```python
from build123d import *

# Parameters (mm, degrees)
RESSALTO_EXTRUS_O1_DEPTH                = 3
BROCA_DE_ROSQUEAR_PARA_TARRAXA_DE_M61_D = 5
ESBO_O4_W                               = 17.804449836
ESBO_O4_H                               = 9.873376728
CORTE_EXTRUS_O1_DEPTH                   = 149.227737241


with BuildPart() as part:
    # Esboço1 → Ressalto-extrusão1 (new body)
    with BuildSketch(Plane.XY):
        Polygon((0, 0), (117.509029813, -27.129097154), (117.509029813, 63.170902846), (0, 90.3), align=None)
    extrude(amount=RESSALTO_EXTRUS_O1_DEPTH)

    # Broca de rosquear para tarraxa de M61 (through all)
    with Locations(Plane.XY.offset(3)):
        with Locations((14.615550972, 71.531172568), (102.893478841, 51.150607044), (70.057207658, 47.44211239), (47.451822155, 52.660976851)):
            Hole(BROCA_DE_ROSQUEAR_PARA_TARRAXA_DE_M61_D / 2)

    # Esboço4 → Corte-extrusão1 (cut, through all)
    with BuildSketch(Plane.XY.offset(3)):
        with Locations((35.932447389, 16.047022475)):
            Rectangle(ESBO_O4_W, ESBO_O4_H)
    extrude(amount=-CORTE_EXTRUS_O1_DEPTH, mode=Mode.SUBTRACT)


solid = part.part
```
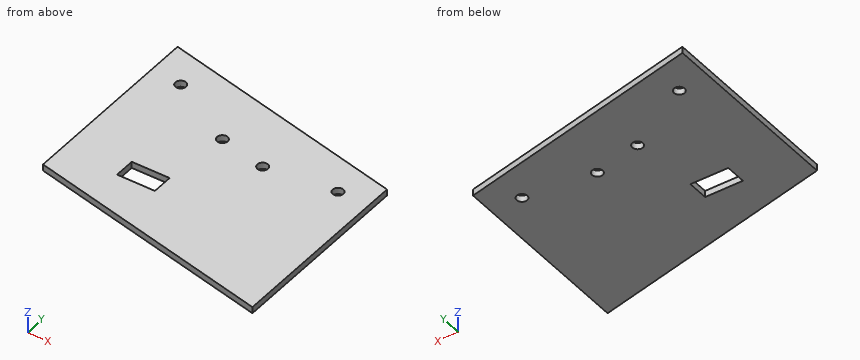
The model under review builds one solid part; all positions refer to its coordinate system, in mm. Round coordinates to 2 decimals unless told otherwise and drop trailing zeros. Write each loop counter-clockwise with the first axis right and the second up, starting at its lowest first coordinate (ties: lowest second). Pieces come first, ordered by that corner, then holes. Notation, with made-up numbers: (37, 4) -> (87, 4) arc R28 ccw to (87, 41) -> close; hole circle Ø9 at (53.25, 12.5). An arc over 180 degrees is marked (long way). Use CSV: the item, a comma, the result in double quotes.
Q1. Consider section A-A (z = 1.2). Give the boundary of the cut face in (x, y), then the cut area to 3 significant figures.
Checks:
outline,"(0, 0) -> (117.51, -27.13) -> (117.51, 63.17) -> (0, 90.3) -> close; hole circle Ø5 at (14.62, 71.53); hole (27.03, 11.11) -> (44.83, 11.11) -> (44.83, 20.98) -> (27.03, 20.98) -> close; hole circle Ø5 at (47.45, 52.66); hole circle Ø5 at (70.06, 47.44); hole circle Ø5 at (102.89, 51.15)"
area,"10,400 mm²"
Q2. Consider section B-B (x = 40.5). Give the boundary of the cut face in (y, z), then the cut area to 3 significant figures.
Checks:
outline,"(-9.35, 0) -> (11.11, 0) -> (11.11, 3) -> (-9.35, 3) -> close; (20.98, 0) -> (80.95, 0) -> (80.95, 3) -> (20.98, 3) -> close"
area,"241 mm²"
Q3. To check wall thickness, follow probe 1 along X at (y, z) = (51.5, 2.7); probe 2 along Y at (x, z) = (32, 1.6); probe 3 along Y at (x, z) = (105, 2.4). State the ranges of each line that lie inside material, in increasing order. Write a range as [from, to].
Checks:
probe 1,"[0, 45.24], [49.67, 100.42], [105.37, 117.51]"
probe 2,"[-7.39, 11.11], [20.98, 82.91]"
probe 3,"[-24.24, 49.8], [52.5, 66.06]"
Q4. For pin 1 Ø1.5 at (x, z) = (34, 1) entering from -Y; pin 2 Ø1 at (x, z) = (54, 1) entering from +Y; pin 3 Ø1.5 at (x, z) = (41.5, 1) entering from -Y, all flat-tipped, find the tip position at first contact; note any pin that passes through.
Checks:
pin 1,"y = -8.02"
pin 2,"y = 77.95"
pin 3,"y = -9.75"
Q5. Consider section D-D (x = 64.5). Give the boundary of the cut face in (y, z).
Checks:
outline,"(-14.89, 0) -> (75.41, 0) -> (75.41, 3) -> (-14.89, 3) -> close"
Q6. Consider section C-C (y = -10.5). Give the boundary of the cut face in (x, z), then the cut area to 3 significant figures.
Checks:
outline,"(45.48, 0) -> (117.51, 0) -> (117.51, 3) -> (45.48, 3) -> close"
area,"216 mm²"
